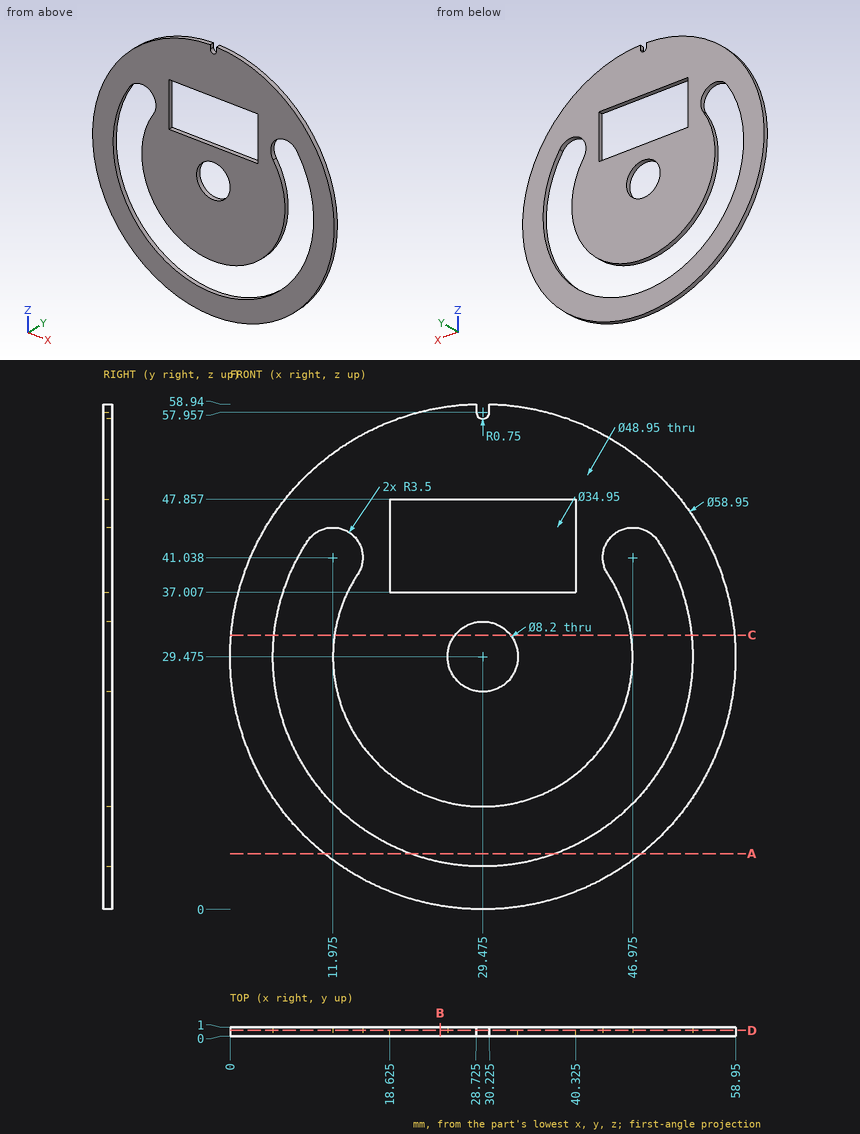
Could you check a few things on this drawing? It's one solid part, dimensions in mm from its lowest x, y, z. Round coordinates to 2 decimals unless told otherwise and drop trailing zeros. Order: outer loops, then holes, each group sorted by start corner. A loop starts at its lowest first (then second) coordinate and runs counter-clockwise, first axis right, second up. Notation, with made-up numbers: M -32.75,-24.5 L 25.25,-24.5 A11 ccw 25.25,-11.5 Z; hole C 45.25,45 d11. An arc over 180 degrees is marked long. One line per question, with ' | ' between items. Start each with the question number.
(1) Suppose I cut it at C-C on z = 32. List the corners of the cut face in (x, y) for me (1 decimal).
(2) For P1, Ø12, axis at x = 50.5, z = 7.5, coming from the +Y side; P2, Ø1, axis at x = 11.5, z = 43.5, coming from the -Y side; P3, Ø0.5, axis at x = 33, y = 0.5, coming from the -Z side, each with a flat end and sliding along its axis, tell me the tip position at first contact or that it passes through.
(3) Suppose I cut it at B-B on x = 24.5. List the corners of the cut face in (y, z) for me.
(4) Please list where these lines run through material, in increasing order: line 1 along Z through (x, y) = (30, 0.1) (1 decimal); line 2 along Z through (x, y) = (22, 0.1) (1 decimal); line 3 along Z through (x, y) = (44, 0.4) (1 decimal).
(5) Suppose I cut it at A-A on z = 6.5. List the corners of the cut face in (x, y) for me.
(6) Suppose I cut it at D-D on y = 0.65. Count the separate pieces of the cut face and the enclosed holes in it, then the cut area to 3 significant figures.
Geometry results:
1) outline: M 0.1,0 L 5.1,0 L 5.1,1 L 0.1,1 Z; M 12.2,0 L 26.2,0 L 26.2,1 L 12.2,1 Z; M 32.7,0 L 46.8,0 L 46.8,1 L 32.7,1 Z; M 53.8,0 L 58.8,0 L 58.8,1 L 53.8,1 Z
2) P1: y = 1 | P2: through | P3: z = 0.18
3) outline: M 0,0.42 L 1,0.42 L 1,5.51 L 0,5.51 Z; M 0,12.72 L 1,12.72 L 1,37.01 L 0,37.01 Z; M 0,47.86 L 1,47.86 L 1,58.53 L 0,58.53 Z
4) line 1: 0 to 5, 12 to 25.4, 33.5 to 37, 47.9 to 57.4 | line 2: 1 to 6.2, 13.7 to 37, 47.9 to 58 | line 3: 3.8 to 9.8, 19.8 to 39.2, 42.9 to 55.1
5) outline: M 11.01,0 L 21.04,0 L 21.04,1 L 11.01,1 Z; M 37.91,0 L 47.94,0 L 47.94,1 L 37.91,1 Z
6) separate pieces: 1 | enclosed holes: 3 | area: 1,770 mm²
